CAD build for the part. Positions are in the model's coordinates, mm. Coordinates: 2 decimals unless noted, no trailing zeros. Order: outer loops, then holes, each group sorted by start corner. A loop starts at its lowest first (then second) coordinate and runs counter-clockwise, first axis right, second up. Notation, with made-up numbers: M 46,32 L 90,32 A21 cw 90,39 Z; hole C -10.5,51 d3. An arc over 180 degrees is marked long. Write item = value, one per line. Start each with the question number.
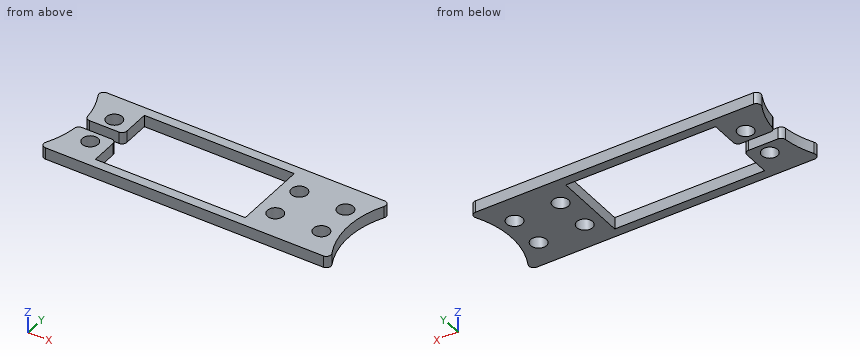
```python
from build123d import *

# Parameters (mm, degrees)
SKETCH1_W           = 40.894
SKETCH1_H           = 20.32
BOSS_EXTRUDE1_DEPTH = 3.2004
SKETCH2_R           = 2.159
CUT_EXTRUDE1_DEPTH  = 3.2004
SKETCH3_W           = 10.481403753
SKETCH3_H           = 3.175
CUT_EXTRUDE2_DEPTH  = 3.2004
FILLET1_R           = 1.27


with BuildPart() as part:
    # Sketch1 → Boss-Extrude1 (new body)
    with BuildSketch(Plane.XY):
        with BuildLine():
            Line((0, 25.4), (80.179895682, 25.4))
            ThreePointArc((80.179895682, 25.4), (76.475447841, 12.7), (80.179895682, 0))
            Line((80.179895682, 0), (0, 0))
            ThreePointArc((0, 0), (3.704447841, 12.7), (0, 25.4))
        make_face()
        with Locations((34.579447813, 12.7)):
            Rectangle(SKETCH1_W, SKETCH1_H, mode=Mode.SUBTRACT)
    extrude(amount=BOSS_EXTRUDE1_DEPTH)

    # Sketch2 → Cut-Extrude1 (cut)
    with BuildSketch(Plane.XY.offset(3.2004)):
        with Locations((9.329447813, 17.7)):
            Circle(SKETCH2_R)
        with Locations((59.829447813, 7.7)):
            Circle(SKETCH2_R)
        with Locations((59.829447813, 17.7)):
            Circle(SKETCH2_R)
        with Locations((9.329447813, 7.7)):
            Circle(SKETCH2_R)
        with Locations((72.404688187, 17.7)):
            Circle(SKETCH2_R)
        with Locations((72.404688187, 7.7)):
            Circle(SKETCH2_R)
    extrude(amount=-CUT_EXTRUDE1_DEPTH, mode=Mode.SUBTRACT)

    # Sketch3 → Cut-Extrude2 (cut)
    with BuildSketch(Plane.XY.offset(3.2004)):
        with Locations((8.891745937, 12.7)):
            Rectangle(SKETCH3_W, SKETCH3_H)
    extrude(amount=-CUT_EXTRUDE2_DEPTH, mode=Mode.SUBTRACT)

    # Fillet1
    fillet1_edges = [part.edges().sort_by_distance(p)[0] for p in [
        (14.132447813, 11.1125, 1.6002),
        (14.132447813, 14.2875, 1.6002),
        (3.65104406, 14.2875, 1.6002),
        (3.65104406, 11.1125, 1.6002),
        (0, 25.4, 1.6002),
        (80.179895682, 25.4, 1.6002),
        (80.179895682, 0, 1.6002),
        (0, 0, 1.6002),
    ]]
    fillet(fillet1_edges, radius=FILLET1_R)


solid = part.part
```
1. Slice it at B-B (y = 3.25). Write the cut outline in (x, z), plus the area to 3 significant figures.
2. Slice it at A-A (x = 49.5). Write the cut outline in (y, z).
3. Probe L1, parallel to Y at x = 50, z = 1.4; L2, parallel to Y at x = 72, z = 2.3; L3, parallel to X at y = 5.75, z = 2.1. List the from-to ranges inside material, lowest first.
4. Slice it at D-D (y = 7.7). Write the cut outline in (x, z), plus the area to 3 significant figures.
5. Slice it at C-C (z = 0.75). Write the cut outline in (x, y).
6. Flat gauge pins, fed straight in: pin 1 (1.6 mm diameter, centred on y = 20.5, z = 1, fed in from +X); pin 2 (4 mm diameter, centred on x = 72.4, y = 17.7, fed in from +Z); pin 3 (1.6 mm diameter, centred on y = 6.5, z = 2, fed in from +X). Where does each tip first touch, or does it go through?
Calculated:
q1.outline = M 1.73,0 L 14.13,0 L 14.13,3.2 L 1.73,3.2 Z; M 55.03,0 L 78.45,0 L 78.45,3.2 L 55.03,3.2 Z
q1.area = 115 mm²
q2.outline = M 0,0 L 2.54,0 L 2.54,3.2 L 0,3.2 Z; M 22.86,0 L 25.4,0 L 25.4,3.2 L 22.86,3.2 Z
q3.L1 = 0 to 2.54, 22.86 to 25.4
q3.L2 = 0 to 5.58, 9.82 to 15.58, 19.82 to 25.4
q3.L3 = 2.66 to 8.4, 10.26 to 14.13, 55.03 to 58.9, 60.76 to 71.48, 73.33 to 77.52
q4.outline = M 3.17,0 L 7.17,0 L 7.17,3.2 L 3.17,3.2 Z; M 11.49,0 L 14.13,0 L 14.13,3.2 L 11.49,3.2 Z; M 55.03,0 L 57.67,0 L 57.67,3.2 L 55.03,3.2 Z; M 61.99,0 L 70.25,0 L 70.25,3.2 L 61.99,3.2 Z; M 74.56,0 L 77.01,0 L 77.01,3.2 L 74.56,3.2 Z
q4.area = 64.0 mm²
q5.outline = M 1.07,1.85 A1.27 ccw 2.2,0 L 77.98,0 A1.27 ccw 79.11,1.85 A23.62 cw 79.11,23.55 A1.27 ccw 77.98,25.4 L 2.2,25.4 A1.27 ccw 1.07,23.55 A23.62 cw 3.55,15.41 A1.27 ccw 4.81,14.29 L 12.86,14.29 A1.27 ccw 14.13,15.56 L 14.13,22.86 L 55.03,22.86 L 55.03,2.54 L 14.13,2.54 L 14.13,9.84 A1.27 ccw 12.86,11.11 L 4.81,11.11 A1.27 ccw 3.55,9.99 A23.62 cw Z; hole C 9.33,7.7 d4.32; hole C 9.33,17.7 d4.32; hole C 59.83,7.7 d4.32; hole C 59.83,17.7 d4.32; hole C 72.4,7.7 d4.32; hole C 72.4,17.7 d4.32
q6.pin_1 = 78.1
q6.pin_2 = through
q6.pin_3 = 77.54
